```python
from build123d import *

# Parameters (mm, degrees)
F1_DEPTH = 259.08
F2_R     = 68.58
F2_R_2   = 46.99
F3_DEPTH = 76.2
F4_R     = 129.53999
F7_DEPTH = 25.4
F8_R     = 25.4
F9_DEPTH = 76.2


# Not quite as in the source:
# - a fillet or chamfer is up to 0.001 mm smaller than in the source, because OpenCascade refuses the exact size


with BuildPart() as f1:
    # F0 (on Front) → F1 (new body)
    with BuildSketch(Plane.XZ):
        Polygon((39.5514294499, 0), (-237.3085705501, 0), (-237.3085705501, -66.04), (77.6796412272, -66.04), (371.0496412272, 442.0917454165), (313.8573235613, 475.1117454165), align=None)
    extrude(amount=F1_DEPTH)

    # F2 (on face) → F3 (join)
    with BuildSketch(Plane(origin=(29.6635720874, 0, -17.1262713298), x_dir=(0, -1, 0), z_dir=(-0.8660254038, 0, 0.5))):
        with Locations((129.54, 438.8475029477)):
            Circle(F2_R)
        with Locations((129.54, 438.8475029477)):
            Circle(F2_R_2, mode=Mode.SUBTRACT)
    extrude(amount=F3_DEPTH)

    # F4 (radius 129.54 in the source; OpenCascade refuses exactly that, so slightly less here)
    f4_edges = [f1.edges().sort_by_distance(p)[0] for p in [
        (342.453482, -259.08, 458.601745),
        (342.453482, 0, 458.601745),
    ]]
    fillet(f4_edges, radius=F4_R)

    # F6 (on offset) → F7 (join, symmetric)
    with BuildSketch(Plane.XZ.offset(129.54)):
        Polygon((136.0714294499, 167.1775439465), (-237.7703315524, 0), (39.5514294499, 0), align=None)
    extrude(amount=F7_DEPTH, both=True)

    # F8 (on face) → F9 (cut)
    with BuildSketch(Plane.XY):
        with Locations((-186.5085705501, -50.8)):
            Circle(F8_R)
        with Locations((-186.5085705501, -208.28)):
            Circle(F8_R)
        with Locations((-11.2485705501, -50.8)):
            Circle(F8_R)
        with Locations((-11.2485705501, -208.28)):
            Circle(F8_R)
    extrude(amount=-F9_DEPTH, mode=Mode.SUBTRACT)


solid = f1.part
```
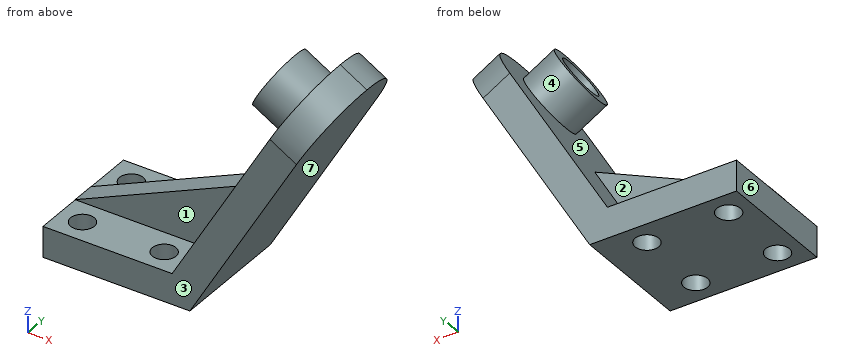
Could you check a few things on this model? Use its own coordinates, in mm. Face numbers are marked on the shaded views. A direction names the side the tool comes from. Coordinates: 2 decimals unless noted, no trailing zeros. Order: outer loops, then holes, each group sorted by start corner. A loop starts at its lowest first (then second) coordinate and runs counter-clockwise, first axis right, second up. Notation, with made-up numbers: M 38,0.5 L 75,0.5 A14 cw 75,15.5 Z; hole C 8.5,39.25 d3. An arc over 180 degrees is marked long. Use one line per item in the form item = value. Start each with the question number.
1. Suppose I cut it at C-C on z = 155. Write out the boundary of the cut face in (x, y).
2. For pin 1 (1 mm diameter, centred on x = 185, y = -165.5, fed in from +Z); pin 2 (12 mm diameter, centred on y = -176, z = 208, fed in from +X); pin 3 (5 mm diameter, centred on x = 187, y = -213.5, fed in from +Z), each with a flat end and sliding along its axis, tell me the tip position at first contact or that it passes through.
3. Suppose I cut it at D-D on y = -165. Write out the boundary of the cut face in (x, z) (3 decimals).
4. Suppose I cut it at A-A on y = -208.28. Write out the boundary of the cut face in (x, z).
5. On a 3-axis mill with a long thin cutter (end or side, diameter ignored), from which of +Z, -Z, +X, -X, +Y, -Y can I reach the whole of each face in a straight line? I mean the marked faces 1, 2 and 3. Say none if no direction works.
6. Please list where these lines run through material, in increasing order: line 1 (X direction, y = -50, z = -16); line 2 (X direction, y = -50, z = -41); line 3 (Z direction, x = -83.5, y = -175).
7. We'd pull the mould along Z, two halves only. Please class the marked faces 4, 5, 6 and 7: +Z half, -Z half, draft (parallel to the pull), parting line (faces both ways), or undercut.
8. Suppose I cut it at B-B on x = 1. Write out the boundary of the cut face in (y, z), then the cut area to 3 significant figures.
Geometry says:
q1.outline = M 108.84,-154.94 L 129.04,-154.94 L 129.04,-259.08 L 205.3,-259.08 L 205.3,0 L 129.04,0 L 129.04,-104.14 L 108.84,-104.14 Z
q2.pin_1 = 365.75
q2.pin_2 = 239.36
q2.pin_3 = 259.72
q3.outline = M -237.309,-66.04 L 77.68,-66.04 L 368.576,437.807 L 311.383,470.827 L 278.438,413.763 L 212.447,451.863 L 198.512,427.729 L 264.504,389.629 L 233.671,336.225 L 167.68,374.325 L 153.746,350.19 L 219.737,312.09 L 39.551,0 L -237.309,0 Z
q4.outline = M -237.31,-66.04 L -211.91,-66.04 L -211.91,0 L -237.31,0 Z; M -161.11,-66.04 L -36.65,-66.04 L -36.65,0 L -161.11,0 Z; M 14.15,-66.04 L 77.68,-66.04 L 357.71,418.99 L 300.52,452.01 L 39.55,0 L 14.15,0 Z
q5.face_1 = +Z, -X, -Y
q5.face_2 = +Z, -X, +Y
q5.face_3 = +Z, -Z, +X, -X, -Y
q6.line_1 = -237.31 to -211.9, -161.12 to -36.64, 14.14 to 106.57
q6.line_2 = -237.31 to -211.9, -161.12 to -36.64, 14.14 to 92.14
q6.line_3 = -66.04 to 0
q7.face_4 = undercut
q7.face_5 = undercut
q7.face_6 = draft
q7.face_7 = -Z half
q8.outline = M -259.08,-66.04 L -230.53,-66.04 L -230.53,0 L -259.08,0 Z; M -186.03,-66.04 L -73.05,-66.04 L -73.05,0 L -104.14,0 L -104.14,106.78 L -154.94,106.78 L -154.94,0 L -186.03,0 Z; M -28.55,-66.04 L 0,-66.04 L 0,0 L -28.55,0 Z
q8.area = 16,700 mm^2
